Here's the drawing with two shaded views (mm, measured from the low corner). I have some questions. Give positions to 0.01 mm unless a question says otherwise; leave off trailing zeros. Order: outer loops, then holes, each group sorted by start corner. A loop starts at its lowest first (then second) coordinate and runs counter-clockwise, first axis right, second up. Notation, with made-up numbers: M -37,47.25 L -10,47.25 A18 ccw -10,71.25 Z; hole C 21.5,-5.5 d7. An arc over 180 degrees is marked long. Write each question's results on one line, items separated by ' | '.
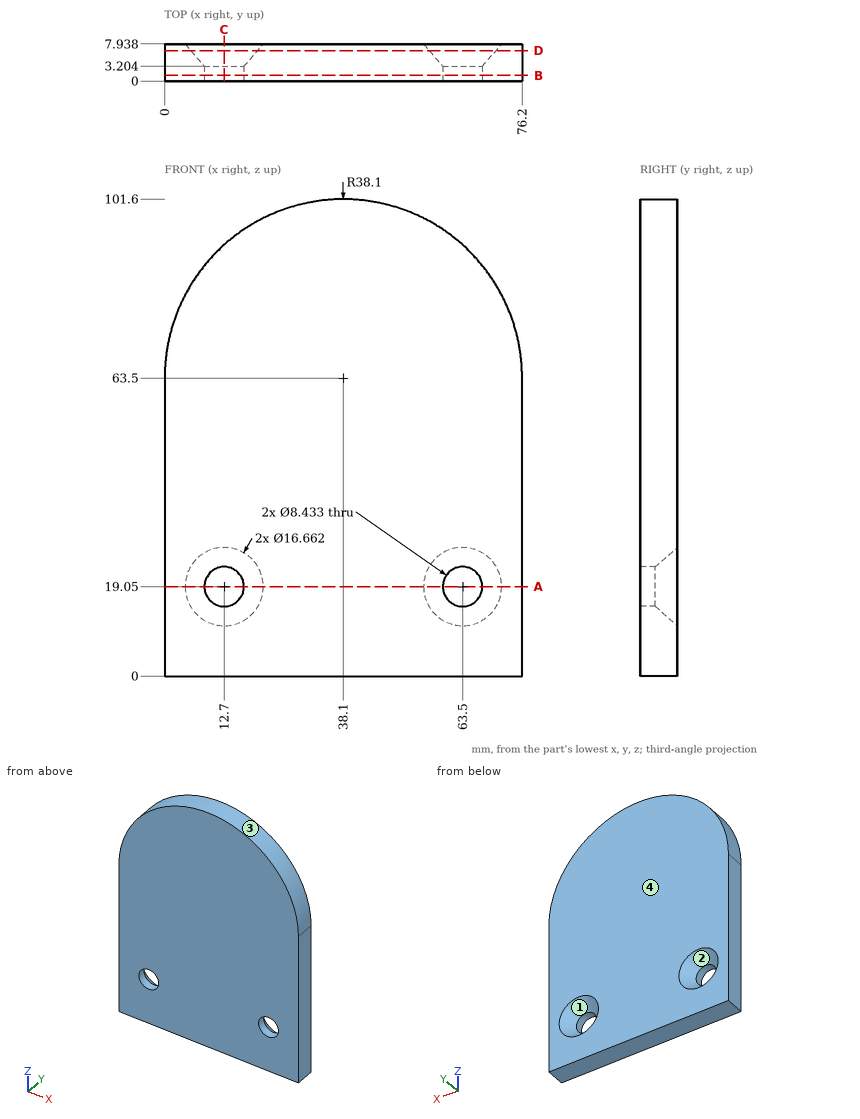
(1) Imagine slicing it at B-B, the plane y = 1.25. Write out the boundary of the cut face in (x, z).
Data:
outline: M 0,0 L 76.2,0 L 76.2,63.5 A38.1 ccw 0,63.5 Z; hole C 12.7,19.05 d8.43; hole C 63.5,19.05 d8.43
(2) Imagine slicing it at C-C, the plane x = 12.7. Write out the boundary of the cut face in (y, z).
Data:
outline: M 0,0 L 7.94,0 L 7.94,10.72 L 3.2,14.83 L 0,14.83 Z; M 0,23.27 L 3.2,23.27 L 7.94,27.38 L 7.94,91.9 L 0,91.9 Z
(3) I need wall thicknesses on L1, parallel to X at y = 1.05, z = 19.05; L2, parallel to X at y = 4, z = 18 (1 decimal); L3, parallel to Z at x = 59.5, y = 4.75 (1 decimal). Which ranges of each line are inside material? Lowest first, please. Write a range as from..to.
Data:
L1: x = 0..8.48, 16.92..59.28, 67.72..76.2 | L2: x = 0..7.9, 17.5..58.7, 68.3..76.2 | L3: z = 0..15.2, 22.9..95
(4) We'd pull the mould along X, two halves only. Please class the marked faces 1, 2, 3 and 4: +X half, -X half, draft (parallel to the pull), parting line (faces both ways), or undercut.
Data:
face 1: undercut | face 2: undercut | face 3: parting line | face 4: draft
(5) Imagine slicing it at D-D, the plane y = 6.5. Write out the boundary of the cut face in (x, z).
Data:
outline: M 0,0 L 76.2,0 L 76.2,63.5 A38.1 ccw 0,63.5 Z; hole C 12.7,19.05 d14.16; hole C 63.5,19.05 d14.16
(6) Imagine slicing it at A-A, the plane z = 19.05. Write out the boundary of the cut face in (x, y), plus the area to 3 significant figures.
Data:
outline: M 0,0 L 8.48,0 L 8.48,3.2 L 4.37,7.94 L 0,7.94 Z; M 16.92,0 L 59.28,0 L 59.28,3.2 L 55.17,7.94 L 21.03,7.94 L 16.92,3.2 Z; M 67.72,0 L 76.2,0 L 76.2,7.94 L 71.83,7.94 L 67.72,3.2 Z | area: 432 mm2
(7) Will this pin go through, and if not, where does the flat tip stop? P1, Ø9.5, axis at x = 12.7, z = 19.05, coming from the +Y side.
Data:
P1: stops at y = 3.82
